Source: CAD feature listing. Evaluate the final solid. Frame: model axes, mm. A direction names the side the tool comes from. Round coordinates to 2 decimals unless told otherwise and drop trailing zeros. Loops run counter-clockwise (first coordinate to the right, second up) from the corner with the lowest first, then second, coordinate; pieces in that order, holes last. Notation, with made-up numbers: M 12,15.25 L 30,15.25 A25 ccw 30,43.25 Z; hole C 65.5,14.25 d11. An arc over 180 degrees is marked long. One line per item, written item: value.
from build123d import *

# Parameters (mm, degrees)
SKETCH2_R                   = 1.35
BOSS_EXTRUDE1_DEPTH         = 4.7625
F_1_4_CLEARANCE_HOLE1_D     = 7.14248
F_1_4_CLEARANCE_HOLE1_DEPTH = 6.35
F_1_4_CLEARANCE_HOLE1_TIP   = 2.145817477
CUT_EXTRUDE1_START          = -4.7625
CUT_EXTRUDE1_DEPTH          = 4.7625


with BuildPart() as part:
    # Sketch2 → Boss-Extrude1 (new body)
    with BuildSketch(Plane.XY):
        with BuildLine():
            Line((-9.2, 12), (9.2, 12))
            ThreePointArc((9.2, 12), (11.321320344, 11.121320344), (12.2, 9))
            Line((12.2, 9), (12.2, -30))
            Line((12.2, -30), (12.2, -35.006033217))
            ThreePointArc((12.2, -35.006033217), (13.381504408, -37.152213482), (15.826842305, -37.301762688))
            ThreePointArc((15.826842305, -37.301762688), (36.936087169, -1.910874265), (12.2, 31.047299132))
            ThreePointArc((12.2, 31.047299132), (0, 33.117218452), (-12.2, 31.047299132))
            ThreePointArc((-12.2, 31.047299132), (-36.936087169, -1.910874265), (-15.826842305, -37.301762688))
            ThreePointArc((-15.826842305, -37.301762688), (-13.381504408, -37.152213482), (-12.2, -35.006033217))
            Line((-12.2, -35.006033217), (-12.2, -30))
            Line((-12.2, -30), (-12.2, 9))
            ThreePointArc((-12.2, 9), (-11.321320344, 11.121320344), (-9.2, 12))
        make_face()
        with Locations(Location((-15, -12.5, 0), (0, 0, 180))):
            Circle(SKETCH2_R, mode=Mode.SUBTRACT)
        with Locations(Location((-15, 4.5, 0), (0, 0, 180))):
            Circle(SKETCH2_R, mode=Mode.SUBTRACT)
        with Locations(Location((-15, -29.5, 0), (0, 0, 180))):
            Circle(SKETCH2_R, mode=Mode.SUBTRACT)
        with Locations(Location((15, -29.5, 0), (0, 0, 180))):
            Circle(SKETCH2_R, mode=Mode.SUBTRACT)
        with Locations(Location((15, -12.5, 0), (0, 0, 180))):
            Circle(SKETCH2_R, mode=Mode.SUBTRACT)
        with Locations(Location((15, 4.5, 0), (0, 0, 180))):
            Circle(SKETCH2_R, mode=Mode.SUBTRACT)
    extrude(amount=BOSS_EXTRUDE1_DEPTH)

    # 1/4 Clearance Hole1
    with Locations(Plane.XY.offset(4.7625)):
        with Locations((-23.371860585, -13.49375), (23.371860585, -13.49375), (0, 26.9875)):
            Hole(F_1_4_CLEARANCE_HOLE1_D / 2, depth=F_1_4_CLEARANCE_HOLE1_DEPTH)
            with Locations((0, 0, -(F_1_4_CLEARANCE_HOLE1_DEPTH + F_1_4_CLEARANCE_HOLE1_TIP / 2))):  # 118° drill point
                Cone(0, F_1_4_CLEARANCE_HOLE1_D / 2, F_1_4_CLEARANCE_HOLE1_TIP, mode=Mode.SUBTRACT)

    # Sketch5 → Cut-Extrude1 (cut)
    with BuildSketch(Plane.XY.offset(4.7625).offset(CUT_EXTRUDE1_START)):
        with BuildLine():
            ThreePointArc((19.800620585, 27.370987986), (18.449246292, 28.187570965), (17.064253254, 28.945736198))
            ThreePointArc((17.064253254, 28.945736198), (19.062973286, 27.075010458), (19.800620585, 24.438654446))
            Line((19.800620585, 24.438654446), (19.800620585, -13.49375))
            ThreePointArc((19.800620585, -13.49375), (23.371860585, -9.92251), (26.943100585, -13.49375))
            Line((26.943100585, -13.49375), (26.943100585, -11.19251))
            ThreePointArc((26.943100585, -11.19251), (27.315074973, -10.294484388), (28.213100585, -9.92251))
            Line((28.213100585, -9.92251), (34.959580577, -9.92251))
            ThreePointArc((34.959580577, -9.92251), (35.94535967, -10.391798079), (36.202612185, -11.45284137))
            ThreePointArc((36.202612185, -11.45284137), (36.354175005, -10.689186113), (36.48963119, -9.92251))
            ThreePointArc((36.48963119, -9.92251), (33.761655161, 11.237661484), (19.800620585, 27.370987986))
        make_face()
        with BuildLine():
            ThreePointArc((-3.57124, 26.9875), (0, 30.55874), (3.57124, 26.9875))
            Line((3.57124, 26.9875), (3.57124, 32.94441106))
            ThreePointArc((3.57124, 32.94441106), (0, 33.117218452), (-3.57124, 32.94441106))
            Line((-3.57124, 32.94441106), (-3.57124, 26.9875))
        make_face()
        with BuildLine():
            ThreePointArc((-19.800620585, 24.438654446), (-19.062973286, 27.075010458), (-17.064253254, 28.945736198))
            ThreePointArc((-17.064253254, 28.945736198), (-18.449246292, 28.187570965), (-19.800620585, 27.370987986))
            ThreePointArc((-19.800620585, 27.370987986), (-33.761655161, 11.237661484), (-36.48963119, -9.92251))
            ThreePointArc((-36.48963119, -9.92251), (-36.354175005, -10.689186113), (-36.202612185, -11.45284137))
            ThreePointArc((-36.202612185, -11.45284137), (-35.94535967, -10.391798079), (-34.959580577, -9.92251))
            Line((-34.959580577, -9.92251), (-28.213100585, -9.92251))
            ThreePointArc((-28.213100585, -9.92251), (-27.315074973, -10.294484388), (-26.943100585, -11.19251))
            Line((-26.943100585, -11.19251), (-26.943100585, -13.49375))
            ThreePointArc((-26.943100585, -13.49375), (-23.371860585, -9.92251), (-19.800620585, -13.49375))
            Line((-19.800620585, -13.49375), (-19.800620585, 24.438654446))
        make_face()
    extrude(amount=CUT_EXTRUDE1_DEPTH, mode=Mode.SUBTRACT)


solid = part.part
1. Pull-direction query (Y, two-part tool) for faces 5 (the face through (-26.943, -12, 2)), 6 (the face through (19.04, 27.11, 2.35)), 7 (the face through (-14.824, -13.839, 2.348)); classes: released by +Y, released by -Y, zero draft, split by the parting line, or undercut.
Report:
face 5: zero draft
face 6: released by +Y
face 7: undercut
2. Ray query, line 1 (X direction, y = 4.5, z = 2.2); line 2 (X direction, y = -11, z = 0.85); line 3 (Y direction, x = 15, z = 2.85). Return the intervals inside material, ascending. Write a range as [from, to].
Report:
line 1: x = [-19.8, -16.35], [-13.65, -12.2], [12.2, 13.65], [16.35, 19.8]
line 2: x = [-36.21, -26.96], [-19.8, -12.2], [12.2, 19.8], [26.96, 36.21]
line 3: y = [-37.53, -30.85], [-28.15, -13.85], [-11.15, 3.15], [5.85, 29.94]
3. Pin query (flat end, axial travel): pin 1 (1.4 mm diameter, centred on x = 31.5, z = 2, fed in from +Y); pin 2 (2.5 mm diameter, centred on y = 13, z = 2, fed in from -X); pin 3 (1 mm diameter, centred on y = 24, z = 2, fed in from +X). Return the tip coordinate at first contact, or that it passes through.
Report:
pin 1: stops at y = -9.92
pin 2: stops at x = -19.8
pin 3: stops at x = 19.8
4. Section query B-B (x = -15). Return the cut outline in (y, z), and give its area (3 significant figures).
Report:
outline: M -37.53,0 L -30.85,0 L -30.85,4.76 L -37.53,4.76 Z; M -28.15,0 L -13.85,0 L -13.85,4.76 L -28.15,4.76 Z; M -11.15,0 L 3.15,0 L 3.15,4.76 L -11.15,4.76 Z; M 5.85,0 L 29.94,0 L 29.94,4.76 L 5.85,4.76 Z
area: 283 mm2
5. Section query C-C (z = 3.7). Count the separate pieces of the cut face and the enclosed holes in it, and give its area (3 significant figures).
Report:
separate pieces: 1
enclosed holes: 6
area: 1,860 mm2
6. Section query D-D (x = 0). Return the cut outline in (y, z), and give its area (3 significant figures).
Report:
outline: M 12,0 L 23.42,0 L 23.42,4.76 L 12,4.76 Z
area: 54.4 mm2
7. Section query A-A (y = 4.5). Return the cut outline in (x, z), and give its area (3 significant figures).
Report:
outline: M -19.8,0 L -16.35,0 L -16.35,4.76 L -19.8,4.76 Z; M -13.65,0 L -12.2,0 L -12.2,4.76 L -13.65,4.76 Z; M 12.2,0 L 13.65,0 L 13.65,4.76 L 12.2,4.76 Z; M 16.35,0 L 19.8,0 L 19.8,4.76 L 16.35,4.76 Z
area: 46.7 mm2
8. Reachability of faces 1 (the face through (3.571, 30, 2)), 2 (the face through (-32, -9.923, 2)), 3 (the face through (0, 12, 2)), 4 (the face through (15.176, -13.839, 2.348)) from +Z, -Z, +X, -X, +Y, -Y: full face, straight path, thin tool, end or side. Return the list, or none.
Report:
face 1: +Z, -Z, +Y
face 2: +Z, -Z, -X, +Y
face 3: +Z, -Z, -Y
face 4: +Z, -Z
